Design review of the part built by this model. Coordinates are the model's own, in mm. A direction names the side the tool comes from. Round coordinates to 2 decimals unless told otherwise and drop trailing zeros. Order: outer loops, then holes, each group sorted by start corner. A loop starts at its lowest first (then second) coordinate and runs counter-clockwise, first axis right, second up. Notation, with made-up numbers: M 24,82.25 L 50,82.25 A15 cw 50,88.25 Z; hole C 85.25,53 d10. An arc over 180 degrees is marked long. Write each question's results on one line, items separated by ' | '. Start each with the question number.
Item 1: Machinability: for faces 5 (the cylindrical face through (-16.5, -0.1, 3.5)), 6 (the flat face through (15, 10, 5.5)), 7 (the flat face through (10.5, 8, 1)), 8 (the flat face through (0, -2.5, 1)), which of the approach directions +Z, -Z, +X, -X, +Y, -Y give a long, thin tool a straight path to every point of the face, cutting with its end or side? Answer none if there is none.
Item 2: Take a section at B-B, the plane z = 2.05. Write out the cut boundary in (x, y).
Item 3: Wall thickness on line 1 (X direction, y = 0, z = 4.1); line 2 (X direction, y = 13.5, z = 1.15); line 3 (Y direction, x = -19.5, z = 2.05): over which ranges is each line inside the solid? List them lowest first. Write a range as [from, to].
Item 4: Clearance check with flat-ended pins moving along their axes: pin 1 (1.2 mm diameter, centred on x = 5.5, z = 1, fed in from +Y); pin 2 (1.5 mm diameter, centred on y = -10.5, z = 1.5, fed in from -X); pin 3 (1.6 mm diameter, centred on y = 11.5, z = 1, fed in from +X). State where each tip first meets the part, or that it passes through.
Item 5: Take a section at A-A, the plane x = 0. Write out the cut boundary in (y, z), plus the area to 3 significant figures.
Item 6: Take a section at D-D, the plane y = -12. Write out the cut boundary in (x, z), plus the area to 3 significant figures.
Item 7: The part is to be moulded in two halves that separate along Y. For faces 1 (the cylindrical face through (19.47, -9.12, 0.88)), 2 (the cylindrical face through (-17.783, 0.541, 2.712)), 3 (the flat face through (0, -1.53, 1)), 4 (the flat face through (-10.5, 8, 1)), say which applies: +Y half, -Y half, draft (parallel to the pull), parting line (faces both ways), or undercut.
Item 8: Take a section at C-C, the plane y = 0. Write out the cut boundary in (x, z).
```python
from build123d import *

# Parameters (mm, degrees)
CYLINDER007_R     = 21.5
CYLINDER007_DEPTH = 10
BOX002_W          = 50
BOX002_H          = 50
BOX002_DEPTH      = 10
CYLINDER006_R     = 1.8
CYLINDER006_DEPTH = 10
CYLINDER005_R     = 3
CYLINDER005_DEPTH = 4
CYLINDER004_R     = 1.8
CYLINDER004_DEPTH = 10
CYLINDER003_R     = 3
CYLINDER003_DEPTH = 4
CYLINDER002_R     = 1.8
CYLINDER002_DEPTH = 10
CYLINDER001_R     = 3
CYLINDER001_DEPTH = 4
BOX001_W          = 23
BOX001_H          = 3.5
BOX001_DEPTH      = 2
BOX_W             = 21
BOX_H             = 25
BOX_DEPTH         = 5
CYLINDER_R        = 21.5
CYLINDER_DEPTH    = 1.5


with BuildPart() as cylinder007:
    # Cylinder007 → Cylinder007 (new body)
    with BuildSketch(Plane.XY):
        Circle(CYLINDER007_R)
    extrude(amount=CYLINDER007_DEPTH)


with BuildPart() as cut005:
    # Box002 → Box002 (new body)
    with BuildSketch(Plane(origin=(-25, -25, 0), x_dir=(1, 0, 0), z_dir=(0, 0, 1))):
        with Locations((25, 25)):
            Rectangle(BOX002_W, BOX002_H)
    extrude(amount=BOX002_DEPTH)

    # Cut005: cut Cylinder007
    add(cylinder007.part, mode=Mode.SUBTRACT)


with BuildPart() as cylinder006:
    # Cylinder006 → Cylinder006 (new body)
    with BuildSketch(Plane(origin=(15.5, 12, -2), x_dir=(1, 0, 0), z_dir=(0, 0, 1))):
        Circle(CYLINDER006_R)
    extrude(amount=CYLINDER006_DEPTH)


with BuildPart() as cylinder005:
    # Cylinder005 → Cylinder005 (new body)
    with BuildSketch(Plane(origin=(15.5, 12, 1.5), x_dir=(1, 0, 0), z_dir=(0, 0, 1))):
        Circle(CYLINDER005_R)
    extrude(amount=CYLINDER005_DEPTH)


with BuildPart() as cylinder004:
    # Cylinder004 → Cylinder004 (new body)
    with BuildSketch(Plane(origin=(15.5, -12, -2), x_dir=(1, 0, 0), z_dir=(0, 0, 1))):
        Circle(CYLINDER004_R)
    extrude(amount=CYLINDER004_DEPTH)


with BuildPart() as cylinder003:
    # Cylinder003 → Cylinder003 (new body)
    with BuildSketch(Plane(origin=(15.5, -12, 1.5), x_dir=(1, 0, 0), z_dir=(0, 0, 1))):
        Circle(CYLINDER003_R)
    extrude(amount=CYLINDER003_DEPTH)


with BuildPart() as cylinder002:
    # Cylinder002 → Cylinder002 (new body)
    with BuildSketch(Plane(origin=(-19.5, 0, -2), x_dir=(1, 0, 0), z_dir=(0, 0, 1))):
        Circle(CYLINDER002_R)
    extrude(amount=CYLINDER002_DEPTH)


with BuildPart() as cylinder001:
    # Cylinder001 → Cylinder001 (new body)
    with BuildSketch(Plane(origin=(-19.5, 0, 1.5), x_dir=(1, 0, 0), z_dir=(0, 0, 1))):
        Circle(CYLINDER001_R)
    extrude(amount=CYLINDER001_DEPTH)


with BuildPart() as box001:
    # Box001 → Box001 (new body)
    with BuildSketch(Plane(origin=(-11.5, -6, 0), x_dir=(1, 0, 0), z_dir=(0, 0, 1))):
        with Locations((11.5, 1.75)):
            Rectangle(BOX001_W, BOX001_H)
    extrude(amount=BOX001_DEPTH)


with BuildPart() as box:
    # Box → Box (new body)
    with BuildSketch(Plane(origin=(-10.5, -1.53, -2), x_dir=(1, 0, 0), z_dir=(0, 0, 1))):
        with Locations((10.5, 12.5)):
            Rectangle(BOX_W, BOX_H)
    extrude(amount=BOX_DEPTH)


with BuildPart() as cut006:
    # Cylinder → Cylinder (new body)
    with BuildSketch(Plane.XY):
        Circle(CYLINDER_R)
    extrude(amount=CYLINDER_DEPTH)

    # Cut: cut Box
    add(box.part, mode=Mode.SUBTRACT)

    # Cut001: cut Box001
    add(box001.part, mode=Mode.SUBTRACT)

    # Fusion: union Cylinder001
    add(cylinder001.part)

    # Cut002: cut Cylinder002
    add(cylinder002.part, mode=Mode.SUBTRACT)

    # Fusion001: union Cylinder003
    add(cylinder003.part)

    # Cut003: cut Cylinder004
    add(cylinder004.part, mode=Mode.SUBTRACT)

    # Fusion002: union Cylinder005
    add(cylinder005.part)

    # Cut004: cut Cylinder006
    add(cylinder006.part, mode=Mode.SUBTRACT)

    # Cut006: cut Cut005
    add(cut005.part, mode=Mode.SUBTRACT)


solid = cut006.part
```
Results list:
1) face 5: +Z | face 6: +Z, +X, -X, +Y, -Y | face 7: +Z, -Z, +Y | face 8: +Z, -Z
2) outline: M -21.37,-2.34 A3 ccw long -21.37,2.34 A21.5 ccw Z; M 15.4,-15 A21.5 ccw 18.38,-11.16 A3 ccw long Z; M 15.4,15 A3 ccw long 18.38,11.16 A21.5 ccw Z; hole C -19.5,0 d3.6; hole C 15.5,-12 d3.6; hole C 15.5,12 d3.6
3) line 1: [-21.5, -21.3], [-17.7, -16.5] | line 2: [-16.73, -10.5], [10.5, 14.51], [16.49, 16.73] | line 3: [-3, -1.8], [1.8, 3]
4) pin 1: y = -1.53 | pin 2: x = -19.16 | pin 3: x = 18.65
5) outline: M -21.5,0 L -6,0 L -6,1.5 L -21.5,1.5 Z; M -2.5,0 L -1.53,0 L -1.53,1.5 L -2.5,1.5 Z | area: 24.7 mm²
6) outline: M -17.84,0 L 13.7,0 L 13.7,5.5 L 12.5,5.5 L 12.5,1.5 L -17.84,1.5 Z; M 17.3,0 L 17.84,0 L 17.84,5.5 L 17.3,5.5 Z | area: 55.1 mm²
7) face 1: parting line | face 2: undercut | face 3: +Y half | face 4: draft
8) outline: M -21.5,0 L -21.3,0 L -21.3,5.5 L -21.5,5.5 Z; M -17.7,0 L -10.5,0 L -10.5,1.5 L -16.5,1.5 L -16.5,5.5 L -17.7,5.5 Z; M 10.5,0 L 21.5,0 L 21.5,1.5 L 10.5,1.5 Z
